Autodesk Fusion 360 part; units mm, degrees
sketch "Sketch1" plane through (0, 0, 0) normal (0, 0, 1) x (1, 0, 0)
  line L0 (15, -35) -> (-15, -35)
  line L1 (-15, -35) -> (-15, 35)
  line L2 (-15, 35) -> (15, 35)
  line L3 (15, 35) -> (15, -35)
  line L4 (15, -35) -> (-15, 35) construction
  line L5 (-15, -35) -> (15, 35) construction
  line L6 (-15, 20) -> (15, 20)
  line L7 (15, 20) -> (15, -20)
  line L8 (15, -20) -> (-15, -20)
  line L9 (-15, -20) -> (-15, 20)
  line L10 (-15, 20) -> (15, -20) construction
  line L11 (15, 20) -> (-15, -20) construction
  line L12 (0, 35) -> (0, 20) construction
  line L13 (0, -20) -> (0, -35) construction
  circle A0 centre (0, -27.5) radius 2.55
  circle A1 centre (0, 27.5) radius 2.55
  dimension "d1" = 30
  dimension "d2" = 15
  dimension "d3" = 40
  dimension "d4" = 5.1
  dimension "d5" = 5.1
extrude "Extrude1" add sketch "Sketch1" along normal blind 5
extrude "Extrude2" add sketch "Sketch1" along normal blind 15 from surface at 5 contours L1 L3 L6 L7 L8 L9
sketch "Sketch2" plane through (15, 0, 0) normal (1, 0, 0) x (0, 0, -1)
  line L0 (0, -35) -> (0, 35)
  line L1 (0, 35) -> (-5, 35)
  line L2 (-5, 35) -> (-5, 20)
  line L3 (-5, 20) -> (-20, 20)
  line L4 (-20, 20) -> (-20, -20)
  line L5 (-20, -20) -> (-5, -20)
  line L6 (-5, -20) -> (-5, -35)
  line L7 (-5, -35) -> (0, -35)
  line L8 (0, 0) -> (-20, 0) construction
  circle A0 centre (-10, 0) radius 4.05
  circle A1 centre (-10, 0) radius 10
  line L9 (-5, 20) -> (-17.3072, 6.8268)
  line L10 (-5, -20) -> (-17.3072, -6.8268)
  dimension "d11" = 8.1
extrude "Extrude3" cut sketch "Sketch2" against normal through all contours A0
extrude "Extrude8" cut sketch "Sketch2" against normal through all contours L3 L4 A1 L9 | L4 L5 A1 L10
fillet "Fillet1" radius 3 4 edges at (-15, 35, 2.5) (15, 35, 2.5) (-15, -35, 2.5) (15, -35, 2.5)
fillet "Fillet1" radius 3 2 edges at (0, 20, 5) (0, -20, 5)
equation "d4 = d5"
Geometry check sheet. Reference: the model listing, model coordinates, mm. A direction names the side the tool comes from. Coordinates: 2 decimals unless noted, no trailing zeros. Loops run counter-clockwise (first coordinate to the right, second up) from the corner with the lowest first, then second, coordinate; pieces in that order, holes last.
Item 1: Release check for a two-part mould opening along X. For faces 1 (the face through (15, 0, 5)), 2 (the face through (-14.1, 34.14, 2.54)), 3 (the face through (-0.33, -30.03, 2.46)) record: released by +X, released by -X, zero draft, split by the parting line, or undercut.
Item 2: Sectioned sample at B-B, the plane z = 1. Record the boundary of the cut face in (x, y).
Item 3: Sectioned sample at A-A, the plane y = -27.5. Record the boundary of the cut face in (x, z), then the cut area to 4 significant figures.
Item 4: Sectioned sample at D-D, the plane z = 13.25. Record the boundary of the cut face in (x, y), then the cut area to 3 significant figures.
Item 5: Access from +Z, -Z, +X, -X, +Y, -Y to the whole of each face (thin tool, end or side, straight path). Record for faces 4 (the face through (0, 35, 2)), 5 (the face through (0, 31, 5)), 6 (the face through (0, -31, 5)).
Item 6: Thickness scan on line 1 (Y direction, x = 0, z = 1.95); line 2 (Z direction, x = -12.5, y = 30); line 3 (Y direction, x = 4.75, z = 8.75). Record the ranges inside material, lowest first.
Item 7: Sectioned sample at C-C, the plane x = 0. Record the boundary of the cut face in (y, z).
Item 8: Go/stop test with flat-tipped pins: pin 1 Ø15 at (x, y) = (5, -25.5) entering from +Z; pin 2 Ø6.5 at (y, z) = (0, 10) entering from +X; pin 3 Ø10 at (y, z) = (-26, 9.5) entering from -X; pin 4 Ø8 at (x, z) = (-5, 17) entering from +Y. Record where each tip stops, or that it passes through.
Check result:
1. face 1: released by +X
1. face 2: released by -X
1. face 3: undercut
2. outline: (-15, -32) arc R3 ccw to (-12, -35) - (12, -35) arc R3 ccw to (15, -32) - (15, 32) arc R3 ccw to (12, 35) - (-12, 35) arc R3 ccw to (-15, 32) - close; hole circle Ø5.1 at (0, -27.5); hole circle Ø5.1 at (0, 27.5)
3. outline: (-15, 0) - (-2.55, 0) - (-2.55, 5) - (-15, 5) - close; (2.55, 0) - (15, 0) - (15, 5) - (2.55, 5) - close
3. area: 124.5 mm2
4. outline: (-15, -11.17) - (15, -11.17) - (15, -2.42) - (-15, -2.42) - close; (-15, 2.42) - (15, 2.42) - (15, 11.17) - (-15, 11.17) - close
4. area: 525 mm2
5. face 4: +Z, -Z, +X, -X, +Y
5. face 5: +Z, +X, -X, +Y
5. face 6: +Z, +X, -X, -Y
6. line 1: y = -35 to -30.05, -24.95 to 24.95, 30.05 to 35
6. line 2: z = 0 to 5
6. line 3: y = -15.99 to -3.85, 3.85 to 15.99
7. outline: (-35, 0) - (-30.05, 0) - (-30.05, 5) - (-35, 5) - close; (-24.95, 0) - (24.95, 0) - (24.95, 5) - (21.18, 5) arc R3 cw to (19.14, 5.81) - (6.83, 17.31) arc R10 ccw to (-6.83, 17.31) - (-19.14, 5.81) arc R3 cw to (-21.18, 5) - (-24.95, 5) - close; (30.05, 0) - (35, 0) - (35, 5) - (30.05, 5) - close; hole circle Ø8.1 at (0, 10)
8. pin 1: stops at z = 6.87
8. pin 2: passes through
8. pin 3: stops at x = -15
8. pin 4: stops at y = 11.44
